```python
from build123d import *

# Parameters (mm, degrees)
SKETCH1_W           = 28.702
SKETCH1_H           = 15.875
BOSS_EXTRUDE1_DEPTH = 10.16
SKETCH2_R           = 1.5875
CUT_EXTRUDE1_DEPTH  = 12.4206
SKETCH4_W           = 0.763653933
SKETCH4_H           = 4.021910712
BOSS_EXTRUDE2_DEPTH = 6.35
SKETCH5_W           = 4.11779101
SKETCH5_H           = 0.870547728
BOSS_EXTRUDE3_DEPTH = 3.048
SKETCH6_W           = 0.83333033
SKETCH6_H           = 4.11779101
BOSS_EXTRUDE4_DEPTH = 3.048
FILLET1_R           = 0.508
SKETCH7_W           = 10.16
SKETCH7_H           = 4.966371196
BOSS_EXTRUDE5_DEPTH = 1.27
SKETCH8_W           = 2.794
SKETCH8_H           = 4.318
BOSS_EXTRUDE6_DEPTH = 2.54
FILLET3_R           = 1.27
FILLET5_R           = 1.27
FILLET6_R           = 1.27


with BuildPart() as part:
    # Sketch1 → Boss-Extrude1 (new body)
    with BuildSketch(Plane.XY):
        with Locations((14.351, 7.9375)):
            Rectangle(SKETCH1_W, SKETCH1_H)
    extrude(amount=BOSS_EXTRUDE1_DEPTH)

    # Sketch2 → Cut-Extrude1 (cut)
    with BuildSketch(Plane.XY.offset(10.16)):
        with Locations((3.683, 13.1318)):
            Circle(SKETCH2_R)
        with Locations((25.908, 2.794)):
            Circle(SKETCH2_R)
    extrude(amount=-CUT_EXTRUDE1_DEPTH, mode=Mode.SUBTRACT)

    # Sketch4 → Boss-Extrude2 (add)
    with BuildSketch(Plane(origin=(0, 0, 0), x_dir=(-1, 0, 0), z_dir=(0, -1, 0))):
        with Locations((-15.348638273, -6.340278275)):
            Rectangle(SKETCH4_W, SKETCH4_H)
    extrude(amount=BOSS_EXTRUDE2_DEPTH)

    # Sketch5 → Boss-Extrude3 (add)
    with BuildSketch(Plane.ZY):
        with Locations((5.992449892, 6.871421324)):
            Rectangle(SKETCH5_W, SKETCH5_H)
    extrude(amount=BOSS_EXTRUDE3_DEPTH)

    # Sketch6 → Boss-Extrude4 (add)
    with BuildSketch(Plane(origin=(0, 6.43614746, 0), x_dir=(-1, 0, 0), z_dir=(0, -1, 0))):
        with Locations((2.631334835, -5.992449892)):
            Rectangle(SKETCH6_W, SKETCH6_H)
    extrude(amount=BOSS_EXTRUDE4_DEPTH)

    # Fillet1
    fillet1_edges = [part.edges().sort_by_distance(p)[0] for p in [
        (-3.048, 7.306695188, 5.992449892),
    ]]
    fillet(fillet1_edges, radius=FILLET1_R)

    # Sketch7 → Boss-Extrude5 (add)
    with BuildSketch(Plane.ZY):
        with Locations((5.08, 8.603517934)):
            Rectangle(SKETCH7_W, SKETCH7_H)
    extrude(amount=BOSS_EXTRUDE5_DEPTH)

    # Sketch8 → Boss-Extrude6 (add)
    with BuildSketch(Plane(origin=(0, 15.875, 0), x_dir=(1, 0, 0), z_dir=(0, 1, 0))):
        with Locations((23.749, -5.461)):
            Rectangle(SKETCH8_W, SKETCH8_H)
    extrude(amount=BOSS_EXTRUDE6_DEPTH)

    # Fillet3
    fillet3_edges = [part.edges().sort_by_distance(p)[0] for p in [
        (22.352, 18.415, 5.461),
        (25.146, 18.415, 5.461),
    ]]
    fillet(fillet3_edges, radius=FILLET3_R)

    # Fillet5
    fillet5_edges = [part.edges().sort_by_distance(p)[0] for p in [
        (0, 15.875, 5.08),
        (28.702, 15.875, 5.08),
        (28.702, 0, 5.08),
        (0, 0, 5.08),
    ]]
    fillet(fillet5_edges, radius=FILLET5_R)

    # Fillet6
    # the kernel refuses this fillet: 1.27 mm, written as the material it takes off along each edge
    with BuildSketch(Plane(origin=(-1.27, 6.120332336, -3.175), x_dir=(1, 0, 0), z_dir=(0, 0, 1))) as fillet6_piece_1_section:
        with BuildLine():
            CenterArc((FILLET6_R, FILLET6_R), FILLET6_R, 180, 90)
            Line((0, FILLET6_R), (0, 0))
            Line((0, 0), (FILLET6_R, 0))
        make_face()
    fillet6_piece_1 = extrude(amount=16.51, mode=Mode.PRIVATE)
    fillet6_piece_1 = split(fillet6_piece_1, bisect_by=Plane(origin=(-0.894827344, 6.253367253, 3.933554387), z_dir=(0, 0, -1)), keep=Keep.TOP, mode=Mode.PRIVATE)
    add(fillet6_piece_1, mode=Mode.SUBTRACT)
    with BuildSketch(Plane(origin=(-1.27, 6.120332336, -3.175), x_dir=(1, 0, 0), z_dir=(0, 0, 1))) as fillet6_piece_2_section:
        with BuildLine():
            CenterArc((FILLET6_R, FILLET6_R), FILLET6_R, 180, 90)
            Line((0, FILLET6_R), (0, 0))
            Line((0, 0), (FILLET6_R, 0))
        make_face()
    fillet6_piece_2 = extrude(amount=16.51, mode=Mode.PRIVATE)
    fillet6_piece_2 = split(fillet6_piece_2, bisect_by=Plane(origin=(-0.894827344, 6.43614746, 5.992449892), z_dir=(0, -1, 0)), keep=Keep.TOP, mode=Mode.PRIVATE)
    add(fillet6_piece_2, mode=Mode.SUBTRACT)
    with BuildSketch(Plane(origin=(-1.27, 6.120332336, -3.175), x_dir=(1, 0, 0), z_dir=(0, 0, 1))) as fillet6_piece_3_section:
        with BuildLine():
            CenterArc((FILLET6_R, FILLET6_R), FILLET6_R, 180, 90)
            Line((0, FILLET6_R), (0, 0))
            Line((0, 0), (FILLET6_R, 0))
        make_face()
    fillet6_piece_3 = extrude(amount=16.51, mode=Mode.PRIVATE)
    fillet6_piece_3 = split(fillet6_piece_3, bisect_by=Plane(origin=(-1.269173055, 7.306695188, 5.992449892), z_dir=(0, 1, 0)), keep=Keep.TOP, mode=Mode.PRIVATE)
    add(fillet6_piece_3, mode=Mode.SUBTRACT)
    with BuildSketch(Plane(origin=(-1.27, 6.120332336, -3.175), x_dir=(1, 0, 0), z_dir=(0, 0, 1))) as fillet6_piece_4_section:
        with BuildLine():
            CenterArc((FILLET6_R, FILLET6_R), FILLET6_R, 180, 90)
            Line((0, FILLET6_R), (0, 0))
            Line((0, 0), (FILLET6_R, 0))
        make_face()
    fillet6_piece_4 = extrude(amount=16.51, mode=Mode.PRIVATE)
    fillet6_piece_4 = split(fillet6_piece_4, bisect_by=Plane(origin=(-1.145263538, 6.665418953, 8.051345397), z_dir=(0, 0, 1)), keep=Keep.TOP, mode=Mode.PRIVATE)
    add(fillet6_piece_4, mode=Mode.SUBTRACT)
    with BuildSketch(Plane(origin=(-1.27, 11.086703532, 13.335), x_dir=(0, -1, 0), z_dir=(0, 0, -1))) as fillet6_piece_5:
        with BuildLine():
            CenterArc((FILLET6_R, -FILLET6_R), FILLET6_R, 90, 90)
            Line((0, -FILLET6_R), (0, 0))
            Line((0, 0), (FILLET6_R, 0))
        make_face()
    extrude(amount=16.51, mode=Mode.SUBTRACT)


solid = part.part
```
Build history of the part. All positions in model axes, mm. A direction names the side the tool comes from. Round coordinates to 2 decimals unless told otherwise and drop trailing zeros. Write each loop counter-clockwise with the first axis right and the second up, starting at its lowest first coordinate (ties: lowest second). Pieces come first, ordered by that corner, then holes.
1) Band-saw the part on D-D, the plane x = 17.5. List the corners of the cut face in (y, z) (3 decimals).
2) Band-saw the part on B-B, the plane z = 6.25. Give the number of separate pieces and of enclosed holes in the cut face, and give its area (3 significant figures).
3) 3-axis set-ups, long thin cutter, end or side, ignore diameter. For faces 1 (the flat face through (-2.6, 3.388, 6)), 2 (the flat face through (-1.27, 9, 5)), 3 (the cylindrical face through (24.784, 18.033, 5.431)), 4 (the flat face through (-2.215, 5, 6)), 5 (the flat face through (28.702, 8, 5)): which of +Z, -Z, +X, -X, +Y, -Y reach the whole face in a straight line?
4) Band-saw the part on A-A, the plane y = 5.5. List the corners of the cut face in (x, z), and give its area (3 significant figures).
5) Band-saw the part on C-C, the plane x = 26. List the corners of the cut face in (y, z) (3 decimals).
6) Drill centre lines: probe 1 along X at (y, z) = (8.5, 8); probe 2 along Y at (x, z) = (22.5, 1.25) (3 decimals); probe 3 along X at (y, z) = (11.75, 2.75). Where is each one in solid material? Low to high.
7) Mould opens along X. For faces 6 (the flat face through (22.352, 16.5, 5.5)), 7 (the cylindrical face through (3.34, 11.58, 5.15)), 8 (the cylindrical face through (28.34, 0.38, 5.15)) say: +X half, -X half, draft (parallel to the pull), parting line (faces both ways), or undercut.
8) Pin check, flat tips, straight feed: pin 1 (1 mm diameter, centred on x = -1.5, z = 5.5, fed in from +Y); pin 2 (1.4 mm diameter, centred on y = 16, z = 6, fed in from -X); pin 3 (0.7 mm diameter, centred on x = -3, z = 7, fed in from -Y). Stop position of each tip, or through.
Ans:
1. outline: (0, 0) - (15.875, 0) - (15.875, 10.16) - (0, 10.16) - close
2. separate pieces: 1
2. enclosed holes: 2
2. area: 459 mm2
3. face 1: +Z, -Z, -X, -Y
3. face 2: +Z, -Z, -X, +Y
3. face 3: +Z, -Z, +X, +Y
3. face 4: +Z, -Z, -Y
3. face 5: +Z, -Z, +X, +Y, -Y
4. outline: (-3.05, 3.93) - (-2.21, 3.93) - (-2.21, 8.05) - (-3.05, 8.05) - close; (0, 0) - (28.7, 0) - (28.7, 10.16) - (0, 10.16) - close
4. area: 295 mm2
5. outline: (0, 0) - (1.209, 0) - (1.209, 10.16) - (0, 10.16) - close; (4.379, 0) - (15.875, 0) - (15.875, 10.16) - (4.379, 10.16) - close
6. probe 1: x = -1.27 to 28.7
6. probe 2: y = 0 to 15.875
6. probe 3: x = 0 to 2.9, 4.46 to 28.7
7. face 6: -X half
7. face 7: undercut
7. face 8: +X half
8. pin 1: stops at y = 10.6
8. pin 2: stops at x = 0.21
8. pin 3: stops at y = 3.39
